Autodesk Inventor part; units mm, degrees
ref_plane "YZ Plane" through (0, 0, 0) normal (1, 0, 0) x (0, 1, 0)
ref_plane "XZ Plane" through (0, 0, 0) normal (0, 1, 0) x (-1, 0, 0)
ref_plane "XY Plane" through (0, 0, 0) normal (0, 0, 1) x (1, 0, 0)
sketch "Sketch1" plane through (0, 0, 0) normal (1, 0, 0) x (0, 1, 0)
  line L0 (0, 0) -> (0, 7) construction
  line L1 (11, 0) -> (11, 7)
  line L2 (11, 7) -> (9, 7)
  line L3 (9, 7) -> (9, 9)
  line L4 (9, 9) -> (14, 9)
  line L5 (11, 0) -> (14, 0)
  arc A0 (14.5851, 7.4744) -> (14, 9) centre (14, 8.125) ccw
  arc A1 (14.5851, 7.4744) -> (14.5851, 1.5256) centre (17.2596, 4.5) ccw
  arc A2 (14, 0) -> (14.5851, 1.5256) centre (14, 0.875) ccw
  line L6 (14.875, 0.875) -> (14.875, -2.7883) construction
  line L7 (13.2596, 4.5) -> (13.2596, 8) construction
  dimension "d0" = 7
  dimension "d1" = 11
  dimension "d2" = 2
  dimension "d3" = 2
  dimension "d5" = 3
  dimension "d6" = 4
  dimension "d7" = 0.875
  dimension "d9" = 13.2596
  dimension "d10" = 14.875
revolve "Revolution1" add sketch "Sketch1" angle 360 about axis through (0, 0, 0) along (0, 0, 1)
properties part number "bearingPulley"
Source: CAD feature listing. Evaluate the final solid. Frame: model axes, mm. A direction names the side the tool comes from. Give positions to 0.01 mm unless a question says otherwise; leave off trailing zeros. Write each loop counter-clockwise with the first axis right and the second up, starting at its lowest first coordinate (ties: lowest second). Pieces come first, ordered by that corner, then holes. Notation, with made-up numbers: M 32.25,45.5 L 74.25,45.5 A27 ccw 74.25,74.5 Z; hole C -5,31.5 d5. An arc over 180 degrees is marked long. Return JSON: item names as keys, results as strings. Group by question number.
1) Pin query (flat end, axial travel): P1, Ø4, axis at x = 10, z = 4, coming from the -Y side; P2, Ø1, axis at y = 8, z = 2.5, coming from the +X side; P3, Ø5, axis at y = 9, z = 8, coming from the -X side. Return the tip coordinate at first contact, or that it passes through.
2) Cut plane D-D, the plane z = 5. Output: boundary loops of the cut face in (x, y).
3) Cut plane A-A, the plane x = 0. Output: boundary loops of the cut face in (y, z) (3 decimals), plus the area to 3 significant figures.
4) Cut plane C-C, the plane z = 2.75. Output: boundary loops of the cut face in (x, y).
5) Set-up query: faces 1 (the face through (-8.923, -1.172, 8.014)), 2 (the face through (10.74, -2.38, 3.55)). Return all of +Z, -Z, +X, -X, +Y, -Y with unobstructed straight access to the full face (end or side cutting, diameter ignored); none if empty.
6) Material intervals for line 1 along Y through (x, z) = (0, 4); line 2 along X through (y, z) = (0, 7.75); line 3 along Y through (x, z) = (0, 8.15), sorted ascending. Write a range as [from, to].
7) Pull-direction query (Y, two-part tool) for faces 3 (the face through (9, 2, 7)), 4 (the face through (9.3, 6.2, 0)); classes: pulls with the +Y half, pulls with the -Y half, needs draft (parallel to the pull), parting line crosses it, or undercut.
Recorded:
{
 "1": {"P1": "stops at y = -10.75", "P2": "stops at x = 11.76", "P3": "stops at x = -13.38"},
 "2": {"outline": "C 0,0 d26.58; hole C 0,0 d22"},
 "3": {"outline": "M -14.585,1.526 A0.875 ccw -14,0 L -11,0 L -11,7 L -9,7 L -9,9 L -14,9 A0.875 ccw -14.585,7.474 A4 cw Z; M 9,7 L 11,7 L 11,0 L 14,0 A0.875 ccw 14.585,1.526 A4 cw 14.585,7.474 A0.875 ccw 14,9 L 9,9 Z", "area": "62.5 mm²"},
 "4": {"outline": "C 0,0 d27.33; hole C 0,0 d22"},
 "5": {"face 1": "+Z, -Z", "face 2": "-Z"},
 "6": {"line 1": "y = [-13.29, -11], [11, 13.29]", "line 2": "x = [-14.79, -9], [9, 14.79]", "line 3": "y = [-14.87, -9], [9, 14.87]"},
 "7": {"face 3": "undercut", "face 4": "needs draft"}
}
